Build history of the part. All positions in model axes, mm. Face numbers are marked on the shaded views. A direction names the side the tool comes from. Round coordinates to 2 decimals unless told otherwise and drop trailing zeros. Loops run counter-clockwise (first coordinate to the right, second up) from the corner with the lowest first, then second, coordinate; pieces in that order, holes last. Notation, with made-up numbers: (67, 72.5) - (99, 72.5) arc R24 cw to (99, 110.5) - close; hole circle Ø8 at (-7.5, 25). An arc over 180 degrees is marked (long way). Put each result on its own line as item: value. Start each with the question number.
from build123d import *

# Parameters (mm, degrees)
F0_R      = 19.05
F1_DEPTH  = 17.272
F2_R      = 3.175
F3_DEPTH  = 10.16
F4_R      = 1.524
F5_DEPTH  = 9.398
F7_R      = 8.255
F8_DEPTH  = 12.446
F9_R      = 17.272
F9_R_2    = 8.89
F10_DEPTH = 15.24
F11_R     = 9.017
F11_R_2   = 8.255
F12_DEPTH = 0.254
F13_R     = 1.905
F14_DEPTH = 5.08
F15_R     = 3.81
F15_R_2   = 1.905
F16_DEPTH = 2.54
F17_R     = 1.905
F18_DEPTH = 14.987
F19_R     = 0.6985
F20_DEPTH = 0.254
F21_R     = 1.778
F22_R     = 1.77799


# Not quite as in the source:
# - a fillet or chamfer is up to 0.001 mm smaller than in the source, because OpenCascade refuses the exact size


with BuildPart() as f1:
    # F0 (on Front) → F1 (new body)
    with BuildSketch(Plane.XZ):
        Circle(F0_R)
    extrude(amount=F1_DEPTH)

    # F2 (on face) → F3 (join)
    with BuildSketch(Plane(origin=(0, 0, 0), x_dir=(-1, 0, 0), z_dir=(0, 1, 0))):
        Circle(F2_R)
    extrude(amount=F3_DEPTH)

    # F4 (on face) → F5 (cut)
    with BuildSketch(Plane(origin=(0, 10.16, 0), x_dir=(-1, 0, 0), z_dir=(0, 1, 0))):
        Circle(F4_R)
    extrude(amount=-F5_DEPTH, mode=Mode.SUBTRACT)

    # F7 (on face) → F8 (cut)
    with BuildSketch(Plane.XZ.offset(17.272)):
        Circle(F7_R)
    extrude(amount=-F8_DEPTH, mode=Mode.SUBTRACT)

    # F9 (on face) → F10 (cut)
    with BuildSketch(Plane(origin=(0, 0, 0), x_dir=(-1, 0, 0), z_dir=(0, 1, 0))):
        Circle(F9_R)
        Circle(F9_R_2, mode=Mode.SUBTRACT)
    extrude(amount=-F10_DEPTH, mode=Mode.SUBTRACT)

    # F11 (on face) → F12 (join)
    with BuildSketch(Plane.XZ.offset(17.272)):
        Circle(F11_R)
        Circle(F11_R_2, mode=Mode.SUBTRACT)
    extrude(amount=F12_DEPTH)

    # F13 (on face) → F14 (join)
    with BuildSketch(Plane.XZ.offset(4.826)):
        Circle(F13_R)
    extrude(amount=F14_DEPTH)

    # F15 (on face) → F16 (join)
    with BuildSketch(Plane.XZ.offset(4.826)):
        Circle(F15_R)
        Circle(F15_R_2, mode=Mode.SUBTRACT)
    extrude(amount=F16_DEPTH)

    # F17 (on face) → F18 (cut, through all)
    with BuildSketch(Plane.XZ.offset(4.826)):
        with Locations((-4.2682749969, 4.2629666667)):
            Circle(F17_R)
        with Locations((0, 6.0325)):
            Circle(F17_R)
        with Locations((4.2629666667, 4.2682749969)):
            Circle(F17_R)
        with Locations((6.0325, 0)):
            Circle(F17_R)
        with Locations((4.2682749969, -4.2629666667)):
            Circle(F17_R)
        with Locations((0, -6.0325)):
            Circle(F17_R)
        with Locations((-4.2629666667, -4.2682749969)):
            Circle(F17_R)
        with Locations((-6.0325, 0)):
            Circle(F17_R)
    extrude(amount=-F18_DEPTH, mode=Mode.SUBTRACT)

    # F19 (on face) → F20 (join)
    with BuildSketch(Plane.XZ.offset(7.366)):
        with Locations((-1.6795963584, 2.3117660614)):
            Circle(F19_R)
        with Locations((0, 2.8575)):
            Circle(F19_R)
        with Locations((1.6795963584, 2.3117660614)):
            Circle(F19_R)
        with Locations((2.7176439953, 0.8830160614)):
            Circle(F19_R)
        with Locations((1.6795963584, -2.3117660614)):
            Circle(F19_R)
        with Locations((0, -2.8575)):
            Circle(F19_R)
        with Locations((2.7176439953, -0.8830160614)):
            Circle(F19_R)
        with Locations((-1.6795963584, -2.3117660614)):
            Circle(F19_R)
        with Locations((-2.7176439953, -0.8830160614)):
            Circle(F19_R)
        with Locations((-2.7176439953, 0.8830160614)):
            Circle(F19_R)
    extrude(amount=F20_DEPTH)

    # F21
    f21_edges = [f1.edges().sort_by_distance(p)[0] for p in [
        (-19.05, -17.272, 0),
    ]]
    fillet(f21_edges, radius=F21_R)

    # F22 (radius 1.778 in the source; OpenCascade refuses exactly that, so slightly less here)
    f22_edges = [f1.edges().sort_by_distance(p)[0] for p in [
        (-19.05, 0, 0),
    ]]
    fillet(f22_edges, radius=F22_R)


solid = f1.part
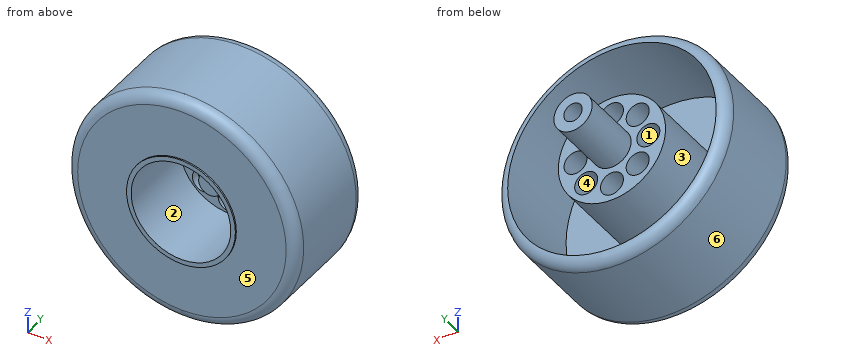
1) Drop flat-ended pins along their axis: pin 1 Ø0.7 at (x, z) = (0, -3) entering from -Y; pin 2 Ø12 at (x, y) = (-11.5, 1.5) entering from +Z; pin 3 Ø4 at (x, z) = (0, 0) entering from -Y. Give the stop position or say it passes through.
2) Which spindle directions (+Z, -Z, +X, -X, +Y, -Y) get a long thin tool onto all of the face, cutting with end or side? Do the marked faces 1, 2 and 3. Say none if no direction does.
3) Pull direction Z, two halves, no side cores. Call the marked faces 4, 5 and 6: pulls with the +Z half, pulls with the -Z half, needs draft (parallel to the pull), parting line crosses it, or undercut.
4) Drill centre lines: line 1 (Z direction, x = 0, y = -10.75) (3 decimals); line 2 (Z direction, x = 0, y = 4.25) (3 decimals); line 3 (X direction, y = -11.25, z = 7.5). Where is each one in solid material? Low to high. Write a range as [from, to].
5) Slice it at A-A, the plane x = 0. State how many separate pieces and enclosed holes the cut face has, and give its area (3 significant figures).
6) Slice it at B-B, the plane y = 3. Write the cut outline in (x, z) (3 decimals).
Taken from the geometry:
1. pin 1: stops at y = -7.62
1. pin 2: stops at z = 17.95
1. pin 3: stops at y = -9.91
2. face 1: +Y, -Y
2. face 2: -Y
2. face 3: +Y
3. face 4: undercut
3. face 5: needs draft
3. face 6: parting line crosses it
4. line 1: z = [-19.05, -17.272], [-8.89, -8.255], [8.255, 8.89], [17.272, 19.05]
4. line 2: z = [-3.175, -1.524], [1.524, 3.175]
4. line 3: x = [-17.51, -15.56], [-4.77, -3.45], [3.45, 4.77], [15.56, 17.51]
5. separate pieces: 3
5. enclosed holes: 0
5. area: 224 mm2
6. outline: circle Ø6.35 at (0, 0); hole circle Ø3.048 at (0, 0)
